Check sheet for the drawn part. Datum: minimum x, y, z corner. Units: mm. Coordinates: 2 decimals unless noted, no trailing zeros. Write each loop counter-clockwise with the first axis right and the second up, starting at its lowest first coordinate (ties: lowest second). Pieces come first, ordered by that corner, then holes. Notation, with made-up numbers: (80, 45.5) - (96, 45.5) arc R23 cw to (96, 70.5) - close; hole circle Ø7 at (56.5, 60.25). An arc over 180 degrees is marked (long way). Use one line per item in the form item = value. Start each with the question number.
1. Cross-section at D-D on x = 43. Record the boundary of the cut face in (y, z), then the cut area to 3 significant figures.
2. Cross-section at C-C on x = 51. Record the boundary of the cut face in (y, z).
3. Cross-section at A-A on y = 2.25. Record the boundary of the cut face in (x, z), then the cut area to 3 significant figures.
4. Cross-section at B-B on z = 62. Record the boundary of the cut face in (x, y).
5. Go/stop test with flat-tipped pins: pin 1 Ø2 at (x, y) = (54.5, 4) entering from +Z; pin 2 Ø1.5 at (x, y) = (50.5, 3.5) entering from +Z; pin 3 Ø1 at (x, y) = (10, 3) entering from -Z (3 decimals). Record where each tip stops, or that it passes through.
6. Draft check along Z on the marked faces 1 and 2. Enter one of: +Z half, -Z half, draft (parallel to the pull), parting line (faces both ways), or undercut.
7. Scan lines: line 1 along Z through (x, y) = (35, 4.55); line 2 along Y through (x, z) = (65.5, 22); line 3 along X through (y, z) = (0.85, 10). Record each from-to range of solid material in increasing order.
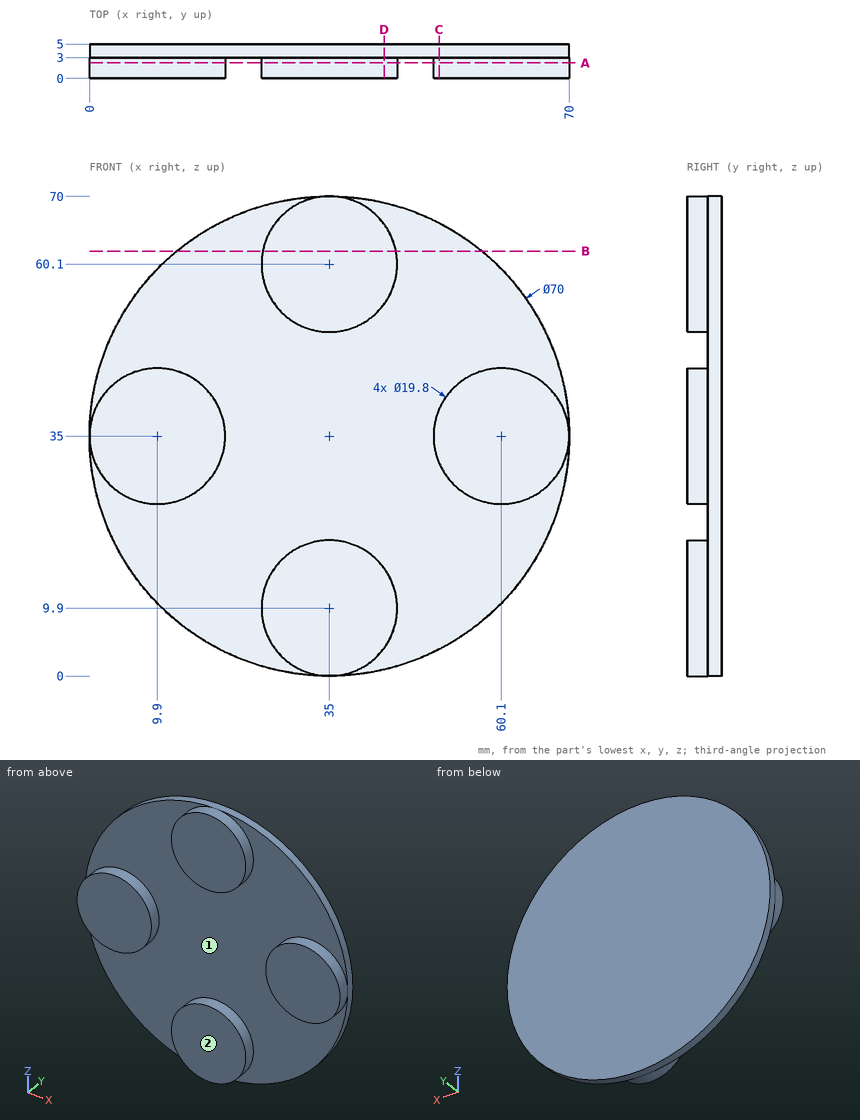
Final values:
q1.outline = (0, 4.07) - (3, 4.07) - (3, 0.93) - (5, 0.93) - (5, 69.07) - (3, 69.07) - (3, 65.93) - (0, 65.93) - (0, 54.27) - (3, 54.27) - (3, 15.73) - (0, 15.73) - close
q1.area = 206 mm²
q2.outline = (0, 31.1) - (3, 31.1) - (3, 3.87) - (5, 3.87) - (5, 66.13) - (3, 66.13) - (3, 38.9) - (0, 38.9) - close
q3.outline = circle Ø19.8 at (9.9, 35); circle Ø19.8 at (35, 9.9); circle Ø19.8 at (35, 60.1); circle Ø19.8 at (60.1, 35)
q3.area = 1,230 mm²
q4.outline = (12.73, 3) - (25.28, 3) - (25.28, 0) - (44.72, 0) - (44.72, 3) - (57.27, 3) - (57.27, 5) - (12.73, 5) - close
q5.pin_1 = 64.71
q5.pin_2 = 66.74
q5.pin_3 = 10.005
q6.face_1 = undercut
q6.face_2 = draft
q7.line_1 = 0 to 70
q7.line_2 = 3 to 5
q7.line_3 = 25.1 to 44.9
